from build123d import *

# Parameters (mm, degrees)
SKETCH1_R           = 13
SKETCH1_W           = 1.8
SKETCH1_H           = 5
SKETCH1_W_2         = 5
SKETCH1_H_2         = 1.8
BOSS_EXTRUDE1_DEPTH = 2
BOSS_EXTRUDE2_DEPTH = 1


with BuildPart() as part:
    # Sketch1 → Boss-Extrude1 (new body)
    with BuildSketch(Plane(origin=(0, 0, 0), x_dir=(1, 0, 0), z_dir=(0, 1, 0))):
        Circle(SKETCH1_R)
        with BuildLine():
            Line((-2.25, 1.58113883), (2.25, 1.58113883))
            ThreePointArc((2.25, 1.58113883), (2.75, 0), (2.25, -1.58113883))
            Line((2.25, -1.58113883), (-2.25, -1.58113883))
            ThreePointArc((-2.25, -1.58113883), (-2.75, 0), (-2.25, 1.58113883))
        make_face(mode=Mode.SUBTRACT)
        Polygon((1.461676593, 7.411039167), (3.006761565, 12.166321749), (4.718663294, 11.610091159), (3.173578322, 6.854808577), align=None, mode=Mode.SUBTRACT)
        with Locations((0, 10)):
            Rectangle(SKETCH1_W, SKETCH1_H, mode=Mode.SUBTRACT)
        Polygon((3.680274097, 6.596634185), (6.619200359, 10.641719157), (8.075430949, 9.583705703), (5.136504687, 5.538620731), align=None, mode=Mode.SUBTRACT)
        Polygon((5.538620731, 5.136504687), (9.583705703, 8.075430949), (10.641719157, 6.619200359), (6.596634185, 3.680274097), align=None, mode=Mode.SUBTRACT)
        Polygon((6.854808577, 3.173578322), (11.610091159, 4.718663294), (12.166321749, 3.006761565), (7.411039167, 1.461676593), align=None, mode=Mode.SUBTRACT)
        with Locations((10, 0)):
            Rectangle(SKETCH1_W_2, SKETCH1_H_2, mode=Mode.SUBTRACT)
        Polygon((7.411039167, -1.461676593), (12.166321749, -3.006761565), (11.610091159, -4.718663294), (6.854808577, -3.173578322), align=None, mode=Mode.SUBTRACT)
        Polygon((6.596634185, -3.680274097), (10.641719157, -6.619200359), (9.583705703, -8.075430949), (5.538620731, -5.136504687), align=None, mode=Mode.SUBTRACT)
        Polygon((5.136504687, -5.538620731), (8.075430949, -9.583705703), (6.619200359, -10.641719157), (3.680274097, -6.596634185), align=None, mode=Mode.SUBTRACT)
        Polygon((3.173578322, -6.854808577), (4.718663294, -11.610091159), (3.006761565, -12.166321749), (1.461676593, -7.411039167), align=None, mode=Mode.SUBTRACT)
        with Locations((0, -10)):
            Rectangle(SKETCH1_W, SKETCH1_H, mode=Mode.SUBTRACT)
        Polygon((-1.461676593, -7.411039167), (-3.006761565, -12.166321749), (-4.718663294, -11.610091159), (-3.173578322, -6.854808577), align=None, mode=Mode.SUBTRACT)
        Polygon((-3.680274097, -6.596634185), (-6.619200359, -10.641719157), (-8.075430949, -9.583705703), (-5.136504687, -5.538620731), align=None, mode=Mode.SUBTRACT)
        Polygon((-5.538620731, -5.136504687), (-9.583705703, -8.075430949), (-10.641719157, -6.619200359), (-6.596634185, -3.680274097), align=None, mode=Mode.SUBTRACT)
        Polygon((-6.854808577, -3.173578322), (-11.610091159, -4.718663294), (-12.166321749, -3.006761565), (-7.411039167, -1.461676593), align=None, mode=Mode.SUBTRACT)
        with Locations((-10, 0)):
            Rectangle(SKETCH1_W_2, SKETCH1_H_2, mode=Mode.SUBTRACT)
        Polygon((-7.411039167, 1.461676593), (-12.166321749, 3.006761565), (-11.610091159, 4.718663294), (-6.854808577, 3.173578322), align=None, mode=Mode.SUBTRACT)
        Polygon((-6.596634185, 3.680274097), (-10.641719157, 6.619200359), (-9.583705703, 8.075430949), (-5.538620731, 5.136504687), align=None, mode=Mode.SUBTRACT)
        Polygon((-5.136504687, 5.538620731), (-8.075430949, 9.583705703), (-6.619200359, 10.641719157), (-3.680274097, 6.596634185), align=None, mode=Mode.SUBTRACT)
        Polygon((-3.173578322, 6.854808577), (-4.718663294, 11.610091159), (-3.006761565, 12.166321749), (-1.461676593, 7.411039167), align=None, mode=Mode.SUBTRACT)
    extrude(amount=BOSS_EXTRUDE1_DEPTH)

    # Sketch2 → Boss-Extrude2 (add)
    with BuildSketch(Plane(origin=(0, 2, 0), x_dir=(1, 0, 0), z_dir=(0, 1, 0))):
        with BuildLine():
            Line((-2.720334968, -2.58113883), (2.720334968, -2.58113883))
            ThreePointArc((2.720334968, -2.58113883), (3.75, 0), (2.720334968, 2.58113883))
            Line((2.720334968, 2.58113883), (-2.720334968, 2.58113883))
            ThreePointArc((-2.720334968, 2.58113883), (-3.75, 0), (-2.720334968, -2.58113883))
        make_face()
        with BuildLine():
            Line((-2.25, -1.58113883), (2.25, -1.58113883))
            ThreePointArc((2.25, -1.58113883), (2.75, 0), (2.25, 1.58113883))
            Line((2.25, 1.58113883), (-2.25, 1.58113883))
            ThreePointArc((-2.25, 1.58113883), (-2.75, 0), (-2.25, -1.58113883))
        make_face(mode=Mode.SUBTRACT)
    extrude(amount=BOSS_EXTRUDE2_DEPTH)


solid = part.part
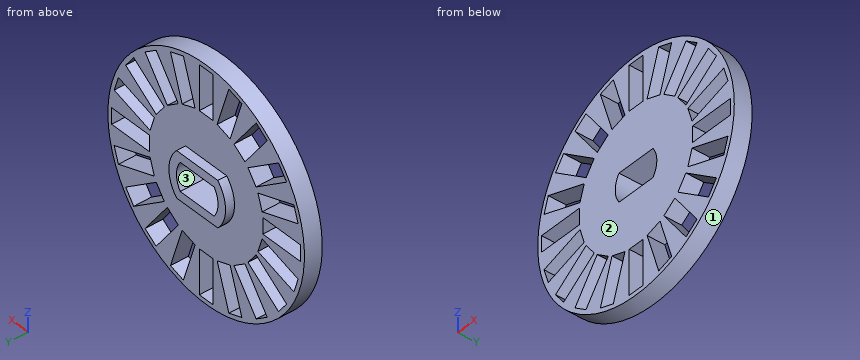
Here's how the part is built. I have some questions about the finished solid (model axes, mm). Face numbers are marked on the shaded views. Coordinates: 2 decimals unless noted, no trailing zeros. Loops run counter-clockwise (first coordinate to the right, second up) from the corner with the lowest first, then second, coordinate; pieces in that order, holes last. Notation, with made-up numbers: (7.5, 32.25) -> (64.5, 32.25) arc R16 ccw to (64.5, 48.25) -> close; hole circle Ø2 at (11.5, 24). An arc over 180 degrees is marked (long way). Use one line per item in the form item = value. Start each with the question number.
(1) Will these pins go through, and if not, where does the flat tip stop? pin 1 (3 mm diameter, centred on x = -5.5, z = 8.5, fed in from +Y); pin 2 (1.6 mm diameter, centred on x = 11, y = 1.5, fed in from +Z); pin 3 (1.6 mm diameter, centred on x = 10.5, y = 1.5, fed in from -Z).
(2) If we section it at C-C (y = 2.7): Please give me the cut outline in (x, z).
(3) Please list where these lines run through material, in increasing order: line 1 along Z through (x, y) = (9.5, 1.75); line 2 along X through (y, z) = (2.05, 0); line 3 along Z through (x, y) = (-1.5, 2.05).
(4) We'd pull the mould along Z, two halves only. Please class the marked faces 1, 2 and 3: pulls with the +Z half, pulls with the -Z half, needs draft (parallel to the pull), parting line crosses it, or undercut.
(5) If we section it at D-D (z = 10): Please give me the cut outline in (x, y), then the cut area to 3 significant figures.
(6) If we section it at A-A (z = 0): Please give me the cut outline in (x, y), then the cut area to 3 significant figures.
(7) If we section it at B-B (x = 0): Please give me the cut outline in (y, z), then the cut area to 3 significant figures.
Verdict:
q1.pin_1 = 2
q1.pin_2 = 8.06
q1.pin_3 = -8.66
q2.outline = (-2.72, -2.58) -> (2.72, -2.58) arc R3.75 ccw to (2.72, 2.58) -> (-2.72, 2.58) arc R3.75 ccw to start; hole (-2.25, -1.58) -> (2.25, -1.58) arc R2.75 ccw to (2.25, 1.58) -> (-2.25, 1.58) arc R2.75 ccw to start
q3.line_1 = -8.87 to -8.01, -5.79 to -4.03, -2.14 to -0.9, 0.9 to 2.14, 4.03 to 5.79, 8.01 to 8.87
q3.line_2 = -3.75 to -2.75, 2.75 to 3.75
q3.line_3 = -2.58 to -1.58, 1.58 to 2.58
q4.face_1 = parting line crosses it
q4.face_2 = needs draft
q4.face_3 = undercut
q5.outline = (-8.31, 0) -> (-7.5, 0) -> (-7.5, 2) -> (-8.31, 2) -> close; (-6.15, 0) -> (-4.2, 0) -> (-4.2, 2) -> (-6.15, 2) -> close; (-2.3, 0) -> (-0.9, 0) -> (-0.9, 2) -> (-2.3, 2) -> close; (0.9, 0) -> (2.3, 0) -> (2.3, 2) -> (0.9, 2) -> close; (4.2, 0) -> (6.15, 0) -> (6.15, 2) -> (4.2, 2) -> close; (7.5, 0) -> (8.31, 0) -> (8.31, 2) -> (7.5, 2) -> close
q5.area = 16.7 mm²
q6.outline = (-13, 0) -> (-12.5, 0) -> (-12.5, 2) -> (-13, 2) -> close; (-7.5, 0) -> (-2.75, 0) -> (-2.75, 3) -> (-3.75, 3) -> (-3.75, 2) -> (-7.5, 2) -> close; (2.75, 0) -> (7.5, 0) -> (7.5, 2) -> (3.75, 2) -> (3.75, 3) -> (2.75, 3) -> close; (12.5, 0) -> (13, 0) -> (13, 2) -> (12.5, 2) -> close
q6.area = 23.0 mm²
q7.outline = (0, -13) -> (2, -13) -> (2, -12.5) -> (0, -12.5) -> close; (0, -7.5) -> (2, -7.5) -> (2, -2.58) -> (3, -2.58) -> (3, -1.58) -> (0, -1.58) -> close; (0, 1.58) -> (3, 1.58) -> (3, 2.58) -> (2, 2.58) -> (2, 7.5) -> (0, 7.5) -> close; (0, 12.5) -> (2, 12.5) -> (2, 13) -> (0, 13) -> close
q7.area = 27.7 mm²
